Could you check a few things on this drawing? It's one solid part, dimensions in mm from its lowest x, y, z. Give positions to 0.01 mm unless a question says otherwise; leave off trailing zeros. Order: outer loops, then holes, each group sorted by start corner. A loop starts at its lowest first (then second) coordinate and runs counter-clockwise, first axis right, second up. Notation, with made-up numbers: (-29.75, 58) - (13.25, 58) arc R17 cw to (13.25, 91) - close; hole circle Ø7 at (-7.75, 70.25). An arc over 180 degrees is marked (long way). Return JSON: item names as keys, results as strings.
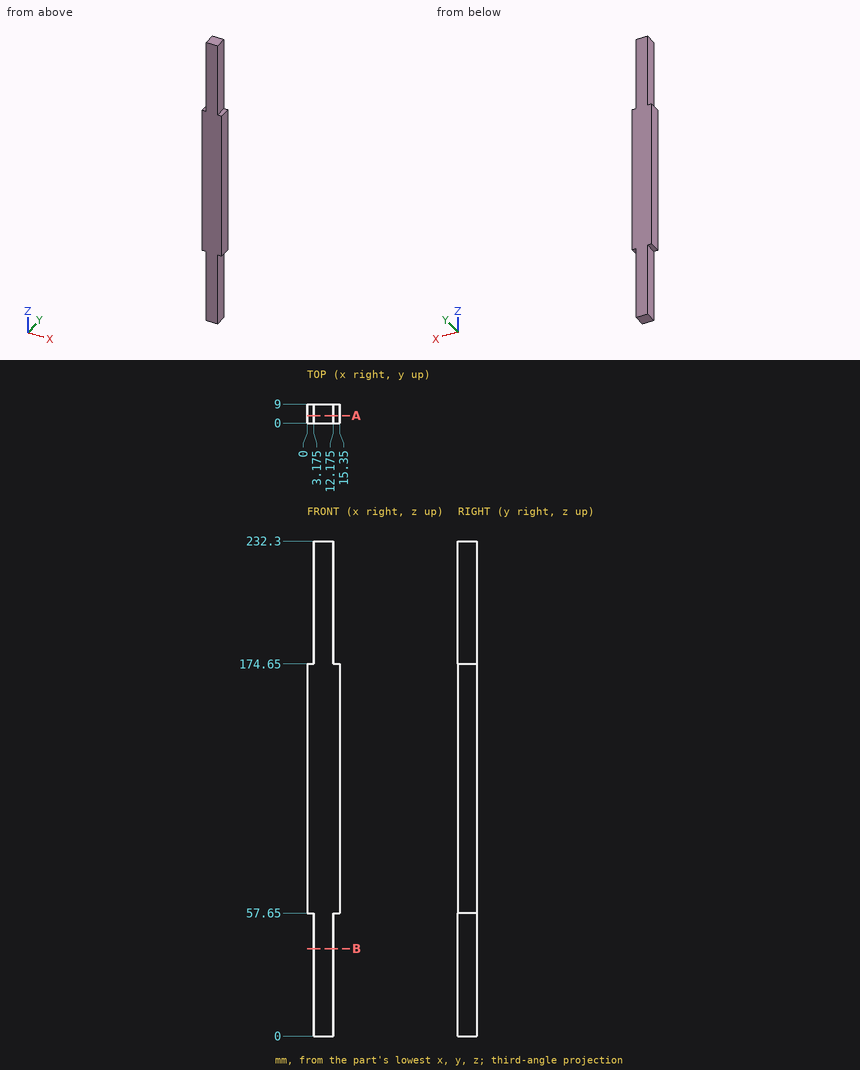
1. Suppose I cut it at A-A (y = 3.5). List the corners of the cut face in (x, z) for me (3 decimals), plus the area to 3 significant figures.
Checks:
{"outline": "(0, 57.65) - (3.175, 57.65) - (3.175, 0) - (12.175, 0) - (12.175, 57.65) - (15.35, 57.65) - (15.35, 174.65) - (12.175, 174.65) - (12.175, 232.3) - (3.175, 232.3) - (3.175, 174.65) - (0, 174.65) - close", "area": "2,830 mm^2"}
2. For pin 1 Ø4.5 at (y, z) = (5.5, 23) entering from +X (3 decimals); pin 2 Ø2.5 at (x, y) = (2, 6) entering from +Z; pin 3 Ø2.5 at (y, z) = (5.5, 211) entering from -X (3 decimals); pin 4 Ø1 at (x, y) = (2, 2) entering from +Z, each with a flat end and sliding along its axis, tell me the tip position at first contact or that it passes through.
Checks:
{"pin 1": "x = 12.175", "pin 2": "z = 232.3", "pin 3": "x = 3.175", "pin 4": "z = 174.65"}
3. If I drill on L1, parallel to Z at x = 14.75, y = 5.5; L2, parallel to X at y = 0.5, z = 37.5 (3 decimals), over which ranges is the centre line in solid material (lowest first)? Write a range as [from, to].
Checks:
{"L1": "[57.65, 174.65]", "L2": "[3.175, 12.175]"}
4. Suppose I cut it at B-B (z = 41). List the corners of the cut face in (x, y) for me (3 decimals), plus the area to 3 significant figures.
Checks:
{"outline": "(3.175, 0) - (12.175, 0) - (12.175, 9) - (3.175, 9) - close", "area": "81.0 mm^2"}
